Read the model definition and answer for the solid it produces. Units are mm, in the model's axes. Face numbers are marked on the shaded views. Round coordinates to 2 decimals unless told otherwise and drop trailing zeros. Order: outer loops, then holes, each group sorted by start corner. A loop starts at its lowest first (then second) coordinate and runs counter-clockwise, first axis right, second up. Notation, with made-up numbers: (-16.5, -13) -> (1.5, -13) arc R17 cw to (1.5, 3) -> close; hole circle Ø1 at (20, -12.5). An arc over 180 degrees is marked (long way). Answer as a JSON object with one key per item and string values. Group by question number.
Item 1: Section C-C, the plane z = 15 is taken. Write down the section's boundary in (x, y), plus the area to 3 significant figures.
Item 2: Consider probe 1 along Z at (x, y) = (0, 49); probe 2 along Y at (x, z) = (75.2, 0); probe 3 along X at (y, z) = (25, -51). Determine where each line is inside the solid, lowest interval first. Write a range as from..to.
Item 3: Given P1, Ø1, axis at x = -13, y = 31, coming from the -Z side; P2, Ø6, axis at x = -30.5, y = 17, coming from the -Z side; P3, Ø3, axis at x = 1, y = 49, coming from the +Z side; P4, Ø3.5, axis at y = 50.8, z = 0, coming from the -X side, each flat-ended and moving along its own axis, determine where each tip first touches the part or whether it passes through.
Item 4: Section B-B, the plane y = 9 is taken. Write down the section's boundary in (x, z) (1 decimal), plus the area to 3 significant figures.
Item 5: Section A-A, the plane x = 0 is taken. Write down the section's boundary in (y, z), plus the area to 3 significant figures.
Item 6: The mould has two halves that part along X. Classify the marked faces 1 and 2: pulls with the +X half, pulls with the -X half, needs draft (parallel to the pull), parting line crosses it, or undercut.
from build123d import *

# Parameters (mm, degrees)
SKETCH1_R               = 75.8825
BOSS_EXTRUDE1_DEPTH     = 63.5
SKETCH2_R               = 73.66
CUT_EXTRUDE1_DEPTH      = 101.6
SKETCH4_R               = 1.5875
CUT_EXTRUDE4_DEPTH      = 76.8825
CUT_EXTRUDE4_DEPTH_BACK = 76.8825


with BuildPart() as part:
    # Sketch1 → Boss-Extrude1 (new body)
    with BuildSketch(Plane(origin=(0, 0, 0), x_dir=(1, 0, 0), z_dir=(0, 1, 0))):
        Circle(SKETCH1_R)
    extrude(amount=BOSS_EXTRUDE1_DEPTH)

    # Sketch2 → Cut-Extrude1 (cut)
    with BuildSketch(Plane(origin=(0, 63.5, 0), x_dir=(1, 0, 0), z_dir=(0, 1, 0))):
        Circle(SKETCH2_R)
    extrude(amount=-CUT_EXTRUDE1_DEPTH, mode=Mode.SUBTRACT)

    # Sketch4 → Cut-Extrude4 (cut, two sides)
    with BuildSketch(Plane(origin=(0, 0, 0), x_dir=(0, 0, -1), z_dir=(1, 0, 0))) as cut_extrude4_sk:
        with Locations((0, 50.8)):
            Circle(SKETCH4_R)
        with Locations((12.7, 50.8)):
            Circle(SKETCH4_R)
    extrude(amount=CUT_EXTRUDE4_DEPTH, mode=Mode.SUBTRACT)
    extrude(cut_extrude4_sk.sketch, amount=-CUT_EXTRUDE4_DEPTH_BACK, mode=Mode.SUBTRACT)


solid = part.part
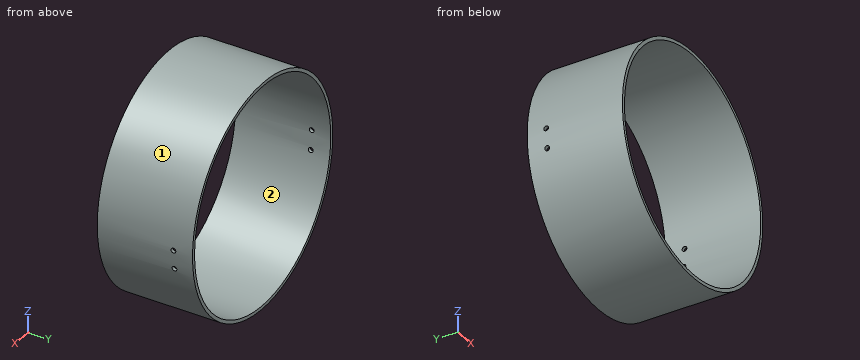
Values found:
{
 "1": {"outline": "(-74.39, 0) -> (-72.12, 0) -> (-72.12, 63.5) -> (-74.39, 63.5) -> close; (72.12, 0) -> (74.39, 0) -> (74.39, 63.5) -> (72.12, 63.5) -> close", "area": "288 mm2"},
 "2": {"probe 1": "-75.88..-73.66, 73.66..75.88", "probe 2": "0..49.21, 52.39..63.5", "probe 3": "-56.19..-53.15, 53.15..56.19"},
 "3": {"P1": "z = -74.85", "P2": "z = -70.72", "P3": "z = 75.88", "P4": "x = -75.88"},
 "4": {"outline": "circle Ø151.8 at (0, 0); hole circle Ø147.3 at (0, 0)", "area": "1,040 mm2"},
 "5": {"outline": "(0, -75.88) -> (63.5, -75.88) -> (63.5, -73.66) -> (0, -73.66) -> close; (0, 73.66) -> (63.5, 73.66) -> (63.5, 75.88) -> (0, 75.88) -> close", "area": "282 mm2"},
 "6": {"face 1": "parting line crosses it", "face 2": "undercut"}
}
